from build123d import *

# Parameters (mm, degrees)
F0_W          = 175
F0_H          = 130
F1_DEPTH      = 15
F1_DEPTH_BACK = 15
F2_W          = 160
F2_H          = 115
F3_DEPTH      = 25
F3_DEPTH_BACK = 25
F4_R          = 15
F5_SIZE       = 3


with BuildPart() as f1:
    # F0 (on Top) → F1 (new body, two sides)
    with BuildSketch(Plane.XY) as f1_sk:
        Rectangle(F0_W, F0_H)
    extrude(amount=F1_DEPTH)
    extrude(f1_sk.sketch, amount=-F1_DEPTH_BACK)

    # F2 (on Top) → F3 (join, two sides)
    with BuildSketch(Plane.XY) as f3_sk:
        with Locations((-7.5, 7.5)):
            Rectangle(F2_W, F2_H)
    extrude(amount=F3_DEPTH)
    extrude(f3_sk.sketch, amount=-F3_DEPTH_BACK)

    # F4
    f4_edges = [f1.edges().sort_by_distance(p)[0] for p in [
        (87.5, -65, 0),
        (72.5, -50, 20),
        (72.5, -50, -20),
    ]]
    fillet(f4_edges, radius=F4_R)

    # F5
    f5_edges = [f1.edges().sort_by_distance(p)[0] for p in [
        (72.5, 15, 25),
        (68.106602, -45.606602, 25),
        (-15, -50, 25),
        (-7.5, -65, 15),
        (72.5, -65, 0),
        (-87.5, -65, 0),
        (-7.5, -65, -15),
        (-15, -50, -25),
        (72.5, 15, -25),
    ]]
    chamfer(f5_edges, length=F5_SIZE)


solid = f1.part
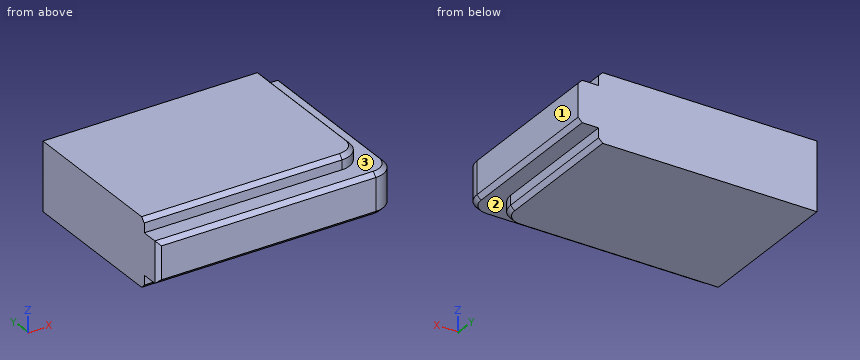
Can you work these out from the model? Positions are in its coordinate system, mm. Face numbers are marked on the shaded views. A direction names the side the tool comes from. Coordinates: 2 decimals unless noted, no trailing zeros. Write each loop counter-clockwise with the first axis right and the second up, starting at its lowest first coordinate (ties: lowest second). Pieces come first, ordered by that corner, then holes. Notation, with made-up numbers: (-36, -1.75) -> (19, -1.75) arc R12 ccw to (19, 3.25) -> close; hole circle Ø8 at (77, -1.5). An arc over 180 degrees is marked (long way). Answer as CSV lines item,"result".
1) If we section it at C-C on z = 18.5: Please give me the cut outline in (x, y), then the cut area to 3 significant figures.
Check result:
outline,"(-87.5, -50) -> (57.5, -50) arc R15 ccw to (72.5, -35) -> (72.5, 65) -> (-87.5, 65) -> close"
area,"18,400 mm²"
2) If I drill on line 1 (X direction, y = -50.5, z = -7); line 2 (X direction, y = 7, z = -19.5); line 3 (Y direction, x = 14, z = 20), over which ranges is the centre line in solid material (lowest first)? Write a range as from..to.
Check result:
line 1,"-87.5..87.49"
line 2,"-87.5..72.5"
line 3,"-50..65"
3) On a 3-axis mill with a long thin cutter (end or side, diameter ignored), from which of +Z, -Z, +X, -X, +Y, -Y can I reach the whole of each face in a straight line? I mean the marked faces 1, 2 and 3. Say none if no direction works.
Check result:
face 1,"+Z, -Z, +X, +Y, -Y"
face 2,"-Z, +X, -Y"
face 3,"+Z, +X, -Y"
4) If we section it at A-A on y = -27: Please give me the cut outline in (x, z).
Check result:
outline,"(-87.5, -25) -> (69.5, -25) -> (72.5, -22) -> (72.5, -15) -> (84.5, -15) -> (87.5, -12) -> (87.5, 12) -> (84.5, 15) -> (72.5, 15) -> (72.5, 22) -> (69.5, 25) -> (-87.5, 25) -> close"
5) Will these pins go through, and if not, where does the flat tip stop? P1, Ø6, axis at x = 68, z = -18.5, coming from the -Y side; P2, Ø5.5, axis at y = -2.5, z = 17.5, coming from the +X side; P3, Ø3.5, axis at x = -35.5, z = -19, coming from the -Y side.
Check result:
P1,"y = -47.99"
P2,"x = 84.75"
P3,"y = -50"
6) If we section it at B-B on x = 12: Please give me the cut outline in (y, z).
Check result:
outline,"(-65, -12) -> (-62, -15) -> (-50, -15) -> (-50, -22) -> (-47, -25) -> (65, -25) -> (65, 25) -> (-47, 25) -> (-50, 22) -> (-50, 15) -> (-62, 15) -> (-65, 12) -> close"
